```python
from build123d import *

# Parameters (mm, degrees)
SKETCH1_W           = 127
SKETCH1_H           = 127
BOSS_EXTRUDE1_DEPTH = 3.175
SKETCH2_R           = 19.05
SKETCH2_R_2         = 1.905
CUT_EXTRUDE1_DEPTH  = 90.858670283


with BuildPart() as part:
    # Sketch1 → Boss-Extrude1 (new body)
    with BuildSketch(Plane(origin=(0, 0, 0), x_dir=(1, 0, 0), z_dir=(0, 1, 0))):
        Rectangle(SKETCH1_W, SKETCH1_H)
    extrude(amount=BOSS_EXTRUDE1_DEPTH)

    # Sketch2 → Cut-Extrude1 (cut, through all)
    with BuildSketch(Plane(origin=(0, 0, 0), x_dir=(1, 0, 0), z_dir=(0, 1, 0))):
        with Locations(Location((0, 0, 0), (0, 0, 270))):
            Circle(SKETCH2_R)
        with Locations(Location((19.05, 31.75, 0), (0, 0, 270))):
            Circle(SKETCH2_R_2)
        with Locations(Location((-19.05, 31.75, 0), (0, 0, 270))):
            Circle(SKETCH2_R_2)
        with Locations(Location((-19.05, -31.75, 0), (0, 0, 270))):
            Circle(SKETCH2_R_2)
        with Locations(Location((19.05, -31.75, 0), (0, 0, 270))):
            Circle(SKETCH2_R_2)
    extrude(amount=CUT_EXTRUDE1_DEPTH, mode=Mode.SUBTRACT)


solid = part.part
```
Check sheet for the modelled part. Datum: model origin and axes. Units: mm. Coordinates: 2 decimals unless noted, no trailing zeros. Write each loop counter-clockwise with the first axis right and the second up, starting at its lowest first coordinate (ties: lowest second). Pieces come first, ordered by that corner, then holes. Notation, with made-up numbers: (41.25, -31) - (46.25, -31) arc R27 ccw to (46.25, -12) - close; hole circle Ø5 at (-3, 37). An arc over 180 degrees is marked (long way). One line per question, with ' | ' between items.
Item 1: Sectioned sample at A-A on z = 31.75. Record the boundary of the cut face in (x, y) (3 decimals), plus the area to 3 significant figures.
Determined:
outline: (-63.5, 0) - (-20.955, 0) - (-20.955, 3.175) - (-63.5, 3.175) - close; (-17.145, 0) - (17.145, 0) - (17.145, 3.175) - (-17.145, 3.175) - close; (20.955, 0) - (63.5, 0) - (63.5, 3.175) - (20.955, 3.175) - close | area: 379 mm2
Item 2: Mould release check, pull along Z, two halves, no side actions. Record for faces 1 (the face through (-1, 2, 63.5)), 2 (the face through (17.89, 1.57, 30.24)), 3 (the face through (-63.5, 2, 1)): pulls with the +Z half, pulls with the -Z half, needs draft (parallel to the pull), parting line crosses it, or undercut.
Determined:
face 1: pulls with the +Z half | face 2: undercut | face 3: needs draft
Item 3: Sectioned sample at D-D on x = -4.5. Record the boundary of the cut face in (y, z) (3 decimals), plus the area to 3 significant figures.
Determined:
outline: (0, -63.5) - (3.175, -63.5) - (3.175, -18.511) - (0, -18.511) - close; (0, 18.511) - (3.175, 18.511) - (3.175, 63.5) - (0, 63.5) - close | area: 286 mm2
Item 4: Sectioned sample at C-C on y = 0.9. Record the boundary of the cut face in (x, z) (3 decimals).
Determined:
outline: (-63.5, -63.5) - (63.5, -63.5) - (63.5, 63.5) - (-63.5, 63.5) - close; hole circle Ø3.81 at (-19.05, -31.75); hole circle Ø3.81 at (-19.05, 31.75); hole circle Ø38.1 at (0, 0); hole circle Ø3.81 at (19.05, -31.75); hole circle Ø3.81 at (19.05, 31.75)
Item 5: Thickness scan on line 1 (X direction, y = 2.05, z = 31.75) (3 decimals); line 2 (X direction, y = 2.55, z = 0); line 3 (Z direction, x = -14.5, y = 0.8). Record the ranges inside material, lowest first. Write a range as [from, to].
Determined:
line 1: x = [-63.5, -20.955], [-17.145, 17.145], [20.955, 63.5] | line 2: x = [-63.5, -19.05], [19.05, 63.5] | line 3: z = [-63.5, -12.36], [12.36, 63.5]
Item 6: Gauge pin test, flat ends, axial feed: P1, Ø6, axis at x = -19.05, z = -31.75, coming from the +Y side (3 decimals); P2, Ø23, axis at x = 0, z = 0, coming from the -Y side. Record the tip position at first contact, or that the pin passes through.
Determined:
P1: stops at y = 3.175 | P2: passes through
Item 7: Sectioned sample at B-B on z = 0. Record the boundary of the cut face in (x, y) (3 decimals).
Determined:
outline: (-63.5, 0) - (-19.05, 0) - (-19.05, 3.175) - (-63.5, 3.175) - close; (19.05, 0) - (63.5, 0) - (63.5, 3.175) - (19.05, 3.175) - close
